Geometry check sheet. Reference: drawing and pictorial views, mm from the part's lowest x, y, z. A direction names the side the tool comes from. Coordinates: 2 decimals unless noted, no trailing zeros. Write each loop counter-clockwise with the first axis right and the second up, starting at its lowest first coordinate (ties: lowest second). Pieces come first, ordered by that corner, then holes. Notation, with made-up numbers: (56, 40) -> (105, 40) arc R30 cw to (105, 79) -> close; hole circle Ø7 at (50, 37.5). An arc over 180 degrees is marked (long way). Answer in a Markdown table with one row per item.
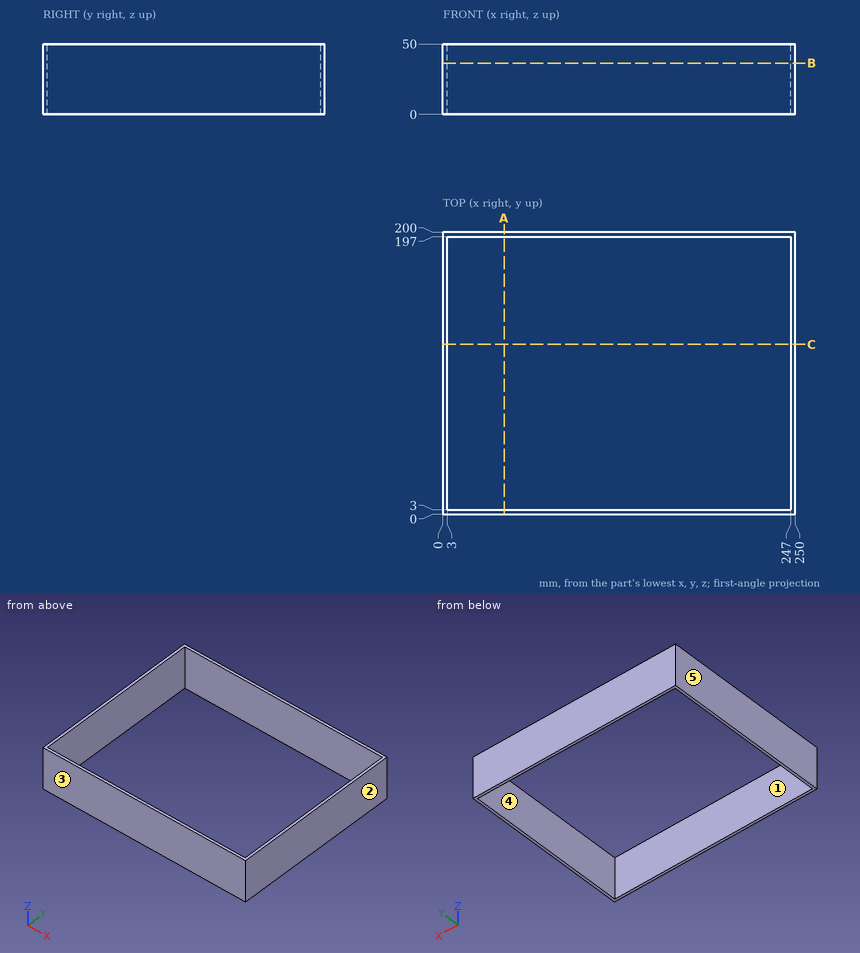
1. Depth check by flat-ended pin: P1, Ø1.5, axis at x = 194, z = 29, coming from the -Y side. Enter the tip coordinate at first touch or a pass-through.
Geometry says:
| item | result |
|---|---|
| P1 | y = 0 |
2. Thickness scan on line 1 (X direction, y = 12, z = 24); line 2 (Y direction, x = 126, z = 44). Record the ranges inside material, lowest first. Write a range as from..to.
Geometry says:
| item | result |
|---|---|
| line 1 | 0..3, 247..250 |
| line 2 | 0..3, 197..200 |
3. Section check C-C, the plane y = 120.5. Record the boundary of the cut face in (x, z).
Geometry says:
| item | result |
|---|---|
| outline | (0, 0) -> (3, 0) -> (3, 50) -> (0, 50) -> close; (247, 0) -> (250, 0) -> (250, 50) -> (247, 50) -> close |
4. Section check B-B, the plane z = 36.5. Record the boundary of the cut face in (x, y), plus the area to 3 significant figures.
Geometry says:
| item | result |
|---|---|
| outline | (0, 0) -> (250, 0) -> (250, 200) -> (0, 200) -> close; hole (3, 3) -> (247, 3) -> (247, 197) -> (3, 197) -> close |
| area | 2,660 mm^2 |
5. Section check A-A, the plane x = 43.5. Record the boundary of the cut face in (y, z), plus the area to 3 significant figures.
Geometry says:
| item | result |
|---|---|
| outline | (0, 0) -> (3, 0) -> (3, 50) -> (0, 50) -> close; (197, 0) -> (200, 0) -> (200, 50) -> (197, 50) -> close |
| area | 300 mm^2 |
6. Tool access check on the marked faces 1 and 2. Record the directions out of +Z, -Z, +X, -X, +Y, -Y that give a thin tool (end or side, any length) a straight path to the whole face; none if there is none.
Geometry says:
| item | result |
|---|---|
| face 1 | +Z, -Z |
| face 2 | +Z, -Z, +X, +Y, -Y |
7. Mould release check, pull along Y, two halves, no side actions. Record for the marked faces 3, 4 and 5: released by +Y, released by -Y, zero draft, split by the parting line, or undercut.
Geometry says:
| item | result |
|---|---|
| face 3 | released by -Y |
| face 4 | undercut |
| face 5 | zero draft |
